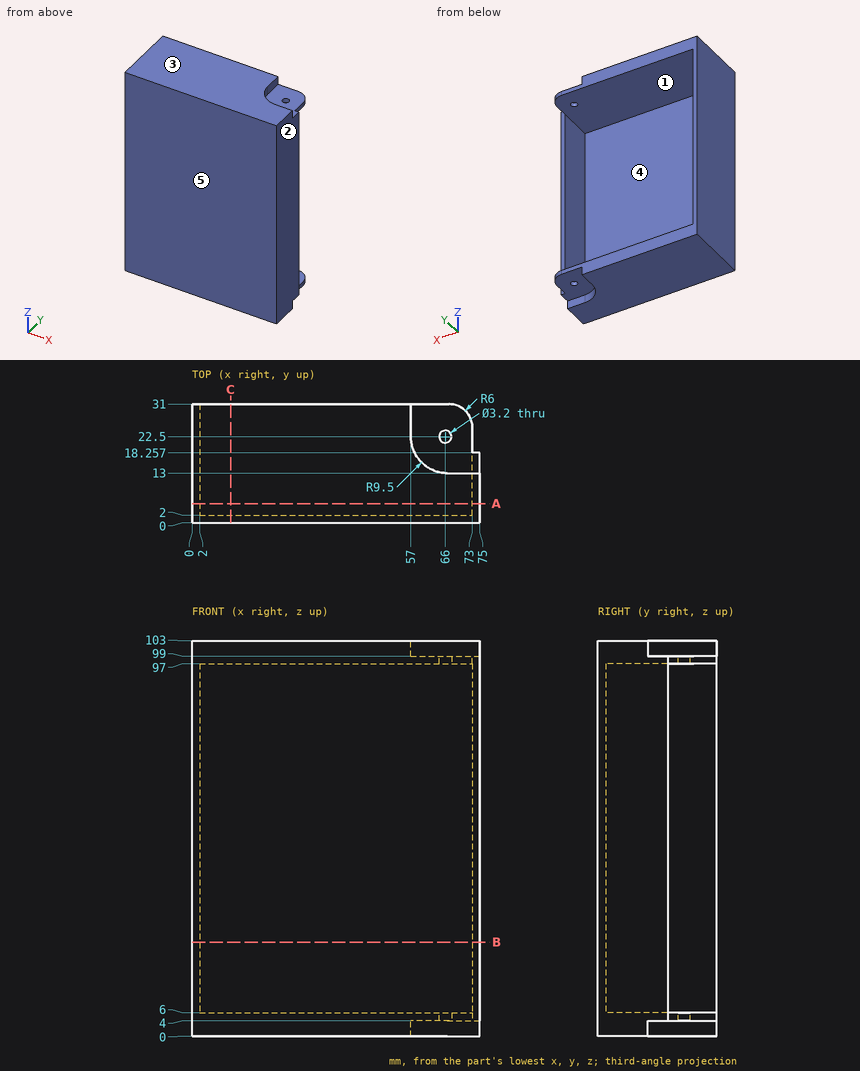
Design review of the part shown in the three views and the two pictorial views. Dimensions are in mm from the part's minimum x, y and z. A direction names the side the tool comes from. Round coordinates to 2 decimals unless told otherwise and drop trailing zeros. Order: outer loops, then holes, each group sorted by start corner. A loop starts at its lowest first (then second) coordinate and runs counter-clockwise, first axis right, second up.
Item 1: Machinability: for the marked faces 4 and 5, which of the approach directions +Z, -Z, +X, -X, +Y, -Y give a long, thin tool a straight path to every point of the face, cutting with its end or side? Answer none if there is none.
Working result:
face 4: +Y
face 5: +Z, -Z, +X, -X, -Y
Item 2: Add section A-A, the plane y = 5. State the section outline as (x, z) points.
Working result:
outline: (0, 0) - (75, 0) - (75, 103) - (0, 103) - close; hole (2, 6) - (73, 6) - (73, 97) - (2, 97) - close
Item 3: Add section C-C, the plane x = 10. State the section outline as (y, z) points.
Working result:
outline: (0, 0) - (31, 0) - (31, 6) - (2, 6) - (2, 97) - (31, 97) - (31, 103) - (0, 103) - close
Item 4: Add section B-B, the plane z = 24.5. State the section outline as (x, y) points.
Working result:
outline: (0, 0) - (75, 0) - (75, 18.26) - (73, 18.26) - (73, 2) - (2, 2) - (2, 31) - (0, 31) - close
Item 5: Draft analysis for pull direction X (two halves, no side actions). For the marked faces 1, 2 and 3, state which applies: released by +X, released by -X, zero draft, split by the parting line, or undercut.
Working result:
face 1: undercut
face 2: released by +X
face 3: zero draft
Item 6: To check wall thickness, follow probe 1 along Z at (x, y) = (57, 14); probe 2 along Y at (x, z) = (66, 98); probe 3 along Z at (x, y) = (68.5, 22.5). State the ranges of each line that lie inside material, in increasing order.
Working result:
probe 1: z = 0 to 6, 97 to 103
probe 2: y = 0 to 20.9, 24.1 to 31
probe 3: z = 4 to 6, 97 to 99
Item 7: For pin 1 (5.5 mm diameter, centred on x = 64.5, y = 18.5, fed in from -Z); pin 2 (2 mm diameter, centred on x = 71, z = 101.5, fed in from +Y); pin 3 (2 mm diameter, centred on x = 74.5, z = 61.5, fed in from +Y); pin 4 (3 mm diameter, centred on x = 66, y = 22.5, fed in from +Z), all flat-tipped, find the tip position at first contact; note any pin that passes through.
Working result:
pin 1: stops at z = 4
pin 2: stops at y = 13
pin 3: stops at y = 18.26
pin 4: passes through
